Input: part model. Units: mm. Frame: model coordinates. A direction names the side the tool comes from. Coordinates: 2 decimals unless noted, no trailing zeros. Write each loop counter-clockwise with the first axis right and the second up, starting at its lowest first coordinate (ties: lowest second). Pieces come first, ordered by that corner, then holes. Notation, with made-up numbers: (83, 86.5) - (118, 86.5) arc R9 cw to (118, 96.5) - close; hole circle Ø11 at (18.5, -34.5). An arc over 180 degrees is marked (long way). Put each result on its own line as item: value. Start each with the question number.
1. Access query for faces 1 (the flat face through (6, 5.556, 0)), 2 (the cylindrical face through (21.68, 3.86, -5.04)), 3 (the flat face through (12.7, -6, 0)). Directions: +Z, -Z, +X, -X, +Y, -Y. A direction counts if a zero-diameter tool reaches every point of the face in a straight line with its end or side. Return the directions, or none.
2. Pin query (flat end, axial travel): pin 1 (2 mm diameter, centred on x = 3.5, z = 3, fed in from -Y); pin 2 (2 mm diameter, centred on x = 10.5, y = 5.5, fed in from +Z); pin 3 (1.9 mm diameter, centred on y = 7, z = -3, fed in from -X). Return the tip coordinate at first contact, or that it passes through.
3. Pull-direction query (Z, two-part tool) for faces 4 (the cylindrical face through (13.77, 1.93, -2.52)), 5 (the cylindrical face through (9.42, -0.35, -7.93)), 6 (the flat face through (6, -5.556, 0)); classes: released by +Z, released by -Z, zero draft, split by the parting line, or undercut.
4. Cut plane D-D, the plane z = -4. Return loops of the section in (x, y).
5. Line query: line 1 (Y direction, x = 19, z = 0) (3 decimals); line 2 (Y direction, x = 13, z = 0) (1 decimal); line 3 (X direction, y = 6.25, z = 4.25). Output: solid intervals per line, ascending.
from build123d import *

# Parameters (mm, degrees)
CUT_EXTRUDE2_START = -12.7
CUT_EXTRUDE2_DEPTH = 12.7


with BuildPart() as part:
    # Sketch1 → Revolve1 (revolve)
    with BuildSketch(Plane.XY, mode=Mode.PRIVATE) as revolve1_sk:
        Polygon((0, 3.175), (0, 7.9375), (15.24, 7.9375), (15.24, 6.35), (27.94, 6.35), (27.94, 3.175), align=None)
    revolve(revolve1_sk.sketch.rotate(Axis((0, 0, 0), (1, 0, 0)), 90), axis=Axis((0, 0, 0), (1, 0, 0)))

    # Sketch2 → Cut-Extrude2 (cut)
    with BuildSketch(Plane.ZY.offset(CUT_EXTRUDE2_START)):
        with BuildLine():
            Line((-5.668508815, 5.55625), (5.668508815, 5.55625))
            ThreePointArc((5.668508815, 5.55625), (0, 7.9375), (-5.668508815, 5.55625))
        make_face()
        with BuildLine():
            Line((-5.668508815, -5.55625), (5.668508815, -5.55625))
            ThreePointArc((5.668508815, -5.55625), (0, -7.9375), (-5.668508815, -5.55625))
        make_face()
    extrude(amount=CUT_EXTRUDE2_DEPTH, mode=Mode.SUBTRACT)


solid = part.part
Report:
1. face 1: +Z, -Z, -X, +Y
1. face 2: +X
1. face 3: +Z, -Z, -X, -Y
2. pin 1: stops at y = -5.56
2. pin 2: stops at z = 6.54
2. pin 3: stops at x = 12.7
3. face 4: undercut
3. face 5: split by the parting line
3. face 6: zero draft
4. outline: (0, -5.56) - (12.7, -5.56) - (12.7, -6.86) - (15.24, -6.86) - (15.24, -4.93) - (27.94, -4.93) - (27.94, 4.93) - (15.24, 4.93) - (15.24, 6.86) - (12.7, 6.86) - (12.7, 5.56) - (0, 5.56) - close
5. line 1: y = -6.35 to -3.175, 3.175 to 6.35
5. line 2: y = -7.9 to -3.2, 3.2 to 7.9
5. line 3: x = 12.7 to 15.24
